Autodesk Inventor part; units mm, degrees
ref_plane "YZ Plane" through (0, 0, 0) normal (1, 0, 0) x (0, 1, 0)
ref_plane "XZ Plane" through (0, 0, 0) normal (0, 1, 0) x (-1, 0, 0)
ref_plane "XY Plane" through (0, 0, 0) normal (0, 0, 1) x (1, 0, 0)
sketch "Эскиз1" plane through (0, 0, 0) normal (0, 0, 1) x (1, 0, 0)
  line L0 (8.75, -1.3) -> (-8.75, -1.3)
  line L1 (-8.75, -1.3) -> (-8.75, 1.3)
  line L2 (-8.75, 1.3) -> (8.75, 1.3)
  line L3 (8.75, 1.3) -> (8.75, -1.3)
  line L4 (8.75, -1.3) -> (-8.75, 1.3) construction
  line L5 (-8.75, -1.3) -> (8.75, 1.3) construction
  line L6 (-8, 7.4) -> (-6.4, 7.4)
  line L7 (-6.4, 7.4) -> (-6.4, 1.3)
  line L8 (-6.4, 1.3) -> (-8, 1.3)
  line L9 (-8, 1.3) -> (-8, 7.4)
  line L10 (-8, 1.3) -> (-7.2, 1.3)
  line L11 (-6.4, -3.2) -> (-8, -3.2)
  line L12 (-6.4, -1.3) -> (-6.4, -3.2)
  line L13 (-8, -3.2) -> (-8, -1.3)
  line L14 (-4, 7.4) -> (-4, 1.3)
  line L15 (-5.6, 1.3) -> (-5.6, 7.4)
  line L16 (-5.6, 7.4) -> (-4, 7.4)
  line L17 (-5.6, -3.2) -> (-5.6, -1.3)
  line L18 (-4, -1.3) -> (-4, -3.2)
  line L19 (-4, -3.2) -> (-5.6, -3.2)
  line L20 (-1.6, 7.4) -> (-1.6, 1.3)
  line L21 (-3.2, 1.3) -> (-3.2, 7.4)
  line L22 (-3.2, 7.4) -> (-1.6, 7.4)
  line L23 (-3.2, -3.2) -> (-3.2, -1.3)
  line L24 (-1.6, -1.3) -> (-1.6, -3.2)
  line L25 (-1.6, -3.2) -> (-3.2, -3.2)
  line L26 (0.8, 7.4) -> (0.8, 1.3)
  line L27 (-0.8, 1.3) -> (-0.8, 7.4)
  line L28 (-0.8, 7.4) -> (0.8, 7.4)
  line L29 (-0.8, -3.2) -> (-0.8, -1.3)
  line L30 (0.8, -1.3) -> (0.8, -3.2)
  line L31 (0.8, -3.2) -> (-0.8, -3.2)
  line L32 (3.2, 7.4) -> (3.2, 1.3)
  line L33 (1.6, 1.3) -> (1.6, 7.4)
  line L34 (1.6, 7.4) -> (3.2, 7.4)
  line L35 (1.6, -3.2) -> (1.6, -1.3)
  line L36 (3.2, -1.3) -> (3.2, -3.2)
  line L37 (3.2, -3.2) -> (1.6, -3.2)
  line L38 (5.6, 7.4) -> (5.6, 1.3)
  line L39 (4, 1.3) -> (4, 7.4)
  line L40 (4, 7.4) -> (5.6, 7.4)
  line L41 (4, -3.2) -> (4, -1.3)
  line L42 (5.6, -1.3) -> (5.6, -3.2)
  line L43 (5.6, -3.2) -> (4, -3.2)
  line L44 (8, 7.4) -> (8, 1.3)
  line L45 (6.4, 1.3) -> (6.4, 7.4)
  line L46 (6.4, 7.4) -> (8, 7.4)
  line L47 (6.4, -3.2) -> (6.4, -1.3)
  line L48 (8, -1.3) -> (8, -3.2)
  line L49 (8, -3.2) -> (6.4, -3.2)
  point P0 (0, 0)
  point P1 (8, -1.3)
  point P2 (6.4, -1.3)
  point P3 (5.6, -1.3)
  point P4 (4, -1.3)
  point P5 (3.2, -1.3)
  point P6 (1.6, -1.3)
  point P7 (0.8, -1.3)
  point P8 (-0.8, -1.3)
  point P9 (-1.6, -1.3)
  point P10 (-3.2, -1.3)
  point P11 (-4, -1.3)
  point P12 (-5.6, -1.3)
  point P13 (-5.6, 1.3)
  point P14 (-4, 1.3)
  point P15 (-3.2, 1.3)
  point P16 (-1.6, 1.3)
  point P17 (-0.8, 1.3)
  point P18 (0.8, 1.3)
  point P19 (6.4, 1.3)
  point P20 (8, 1.3)
  point P21 (1.6, 1.3)
  point P22 (3.2, 1.3)
  point P23 (4, 1.3)
  point P24 (5.6, 1.3)
  point P25 (-6.4, 1.3)
  dimension "d0" = 17.5
  dimension "d1" = 2.6
  dimension "d3" = 8.7
  dimension "d7" = 4.5
  dimension "d8" = 0.75
  dimension "d9" = 1.6
  dimension "d12" = 2.4
extrude "Выдавливание1" add sketch "Эскиз1" against normal mid plane 2.6 contours L0 L1 L2 L3
extrude "Выдавливание2" add sketch "Эскиз1" along normal mid plane 1.6 contours L48 L49 L47 L0 | L2 L45 L46 L44 | L42 L43 L41 L0 | L2 L39 L40 L38 | L36 L37 L35 L0 | L2 L33 L34 L32 | L30 L31 L29 L0 | L2 L27 L28 L26 | L24 L25 L23 L0 | L2 L21 L22 L20 | L18 L19 L17 L0 | L2 L15 L16 L14 | L12 L11 L13 L0 | L2 L9 L6 L7
properties part number "ЛЦМК.00002.00.00.00.00.01-01"
Verification items for the finished model (mm, model axes). A direction names the side the tool comes from. Give positions to 0.01 mm unless a question says otherwise; leave off trailing zeros. Order: outer loops, then holes, each group sorted by start corner. A loop starts at its lowest first (then second) coordinate and runs counter-clockwise, first axis right, second up. Notation, with made-up numbers: M -10.75,60 L 2.25,60 A16 cw 2.25,72 Z; hole C -34,-15.75 d9. An arc over 180 degrees is marked long. Answer in a Markdown table with one row per item. Add a question column.
Item 1: Section check C-C, the plane z = 1. Enter the section's corners in (x, y).
Item 2: Section check A-A, the plane y = 2. Enter the section's corners in (x, z).
Item 3: Section check B-B, the plane x = -2. Enter the section's corners in (y, z).
Item 4: Tool access check on faces 4 (the flat face through (0, 4, 0.8)), 5 (the flat face through (8, -2, 0)), 6 (the flat face through (-7, 4, -0.8)), 7 (the flat face through (1.6, 4, 0)). Record the directions out of +Z, -Z, +X, -X, +Y, -Y that give a thin tool (end or side, any length) a straight path to the whole face; none if there is none.
Item 5: Scan lines: probe 1 along Y at (x, z) = (-7, 0.9); probe 2 along Z at (x, y) = (7.25, 2). Record each from-to range of solid material in increasing order. Write a range as from..to.
Item 6: Gauge pin test, flat ends, axial feed: pin 1 (1.3 mm diameter, centred on y = -2, z = 0, fed in from +X); pin 2 (3 mm diameter, centred on x = 6, y = 6, fed in from +Z); pin 3 (0.8 mm diameter, centred on x = -0.5, y = 5.5, fed in from -Z); pin 4 (1.5 mm diameter, centred on y = 2, z = 1, fed in from -X). Record the tip position at first contact, or that the pin passes through.
Item 7: Mould release check, pull along X, two halves, no side actions. Record for faces 1 (the flat face through (8.75, 0, 0)), 2 (the flat face through (2, -2, 0.8)), 3 (the flat face through (6.4, 4, 0)): released by +X, released by -X, zero draft, split by the parting line, or undercut.
Filled sheet:
| question | item | result |
|---|---|---|
| 1 | outline | M -8.75,-1.3 L 8.75,-1.3 L 8.75,1.3 L -8.75,1.3 Z |
| 2 | outline | M -8,-0.8 L -6.4,-0.8 L -6.4,0.8 L -8,0.8 Z; M -5.6,-0.8 L -4,-0.8 L -4,0.8 L -5.6,0.8 Z; M -3.2,-0.8 L -1.6,-0.8 L -1.6,0.8 L -3.2,0.8 Z; M -0.8,-0.8 L 0.8,-0.8 L 0.8,0.8 L -0.8,0.8 Z; M 1.6,-0.8 L 3.2,-0.8 L 3.2,0.8 L 1.6,0.8 Z; M 4,-0.8 L 5.6,-0.8 L 5.6,0.8 L 4,0.8 Z; M 6.4,-0.8 L 8,-0.8 L 8,0.8 L 6.4,0.8 Z |
| 3 | outline | M -3.2,-0.8 L -1.3,-0.8 L -1.3,-1.3 L 1.3,-1.3 L 1.3,-0.8 L 7.4,-0.8 L 7.4,0.8 L 1.3,0.8 L 1.3,1.3 L -1.3,1.3 L -1.3,0.8 L -3.2,0.8 Z |
| 4 | face 4 | +Z, +X, -X, +Y |
| 4 | face 5 | +Z, -Z, +X, -Y |
| 4 | face 6 | -Z, +X, -X, +Y |
| 4 | face 7 | +Z, -Z, +Y |
| 5 | probe 1 | y = -1.3..1.3 |
| 5 | probe 2 | z = -0.8..0.8 |
| 6 | pin 1 | stops at x = 8 |
| 6 | pin 2 | stops at z = 0.8 |
| 6 | pin 3 | stops at z = -0.8 |
| 6 | pin 4 | stops at x = -8.75 |
| 7 | face 1 | released by +X |
| 7 | face 2 | zero draft |
| 7 | face 3 | undercut |
